Work out the finished part from the listing and answer in its coordinate system (mm). A direction names the side the tool comes from. Round coordinates to 2 decimals unless told otherwise and drop trailing zeros. Loops run counter-clockwise (first coordinate to the right, second up) from the corner with the lowest first, then second, coordinate; pieces in that order, holes last.
from build123d import *

# Parameters (mm, degrees)
SALIENTE_EXTRUIR1_DEPTH = 7
SALIENTE_EXTRUIR2_DEPTH = 30
CORTAR_EXTRUIR3_REACH   = 108.292
CROQUIS3_W              = 3
CROQUIS3_H              = 30
CORTAR_EXTRUIR4_DEPTH   = 7
CROQUIS5_R              = 2
CORTAR_EXTRUIR5_DEPTH   = 5


with BuildPart() as part:
    # Croquis1 → Saliente-Extruir1 (new body)
    with BuildSketch(Plane.XY):
        Polygon((-42.5, 52), (-34.5, 52), (-34.5, 44), (-22.5, 44), (-22.5, 36), (22.5, 36), (22.5, 44), (34.5, 44), (34.5, 52), (42.5, 52), (42.5, -48), (-42.5, -48), align=None)
    extrude(amount=SALIENTE_EXTRUIR1_DEPTH)

    # Croquis2 → Saliente-Extruir2 (add)
    with BuildSketch(Plane.XY.offset(7)):
        Polygon((-42.5, 52), (-42.5, -48), (-34.5, -48), (-34.5, 20), (34.5, 20), (34.5, -48), (42.5, -48), (42.5, 52), (34.5, 52), (34.5, 25), (-34.5, 25), (-34.5, 52), align=None)
    extrude(amount=SALIENTE_EXTRUIR2_DEPTH)

    # Cortar-Extruir3: up to this face of the body (flat: up to its plane)
    cortar_extruir3_end = Plane(part.part.faces().sort_by_distance((42.5, 2, 18.5))[0])
    # Croquis3 → Cortar-Extruir3 (cut, up to the picked face)
    with BuildSketch(Plane.ZY.offset(42.5), mode=Mode.PRIVATE) as cortar_extruir3_sk1:
        with BuildLine():
            Line((37, 52), (7, 52))
            add(Edge.make_bspline(
                [(7, 52), (17.9721482, 28.003586462), (37, 25)],
                knots=[0, 0, 0, 0.777512114, 0.777512114, 0.777512114], degree=2))
            Line((37, 25), (37, 52))
        make_face()
    cortar_extruir3_tool1 = split(extrude(cortar_extruir3_sk1.sketch, amount=-CORTAR_EXTRUIR3_REACH, mode=Mode.PRIVATE), bisect_by=cortar_extruir3_end, keep=Keep.BOTH, mode=Mode.PRIVATE)
    # Croquis3 → Cortar-Extruir3 (cut, up to the picked face)
    with BuildSketch(Plane.ZY.offset(42.5), mode=Mode.PRIVATE) as cortar_extruir3_sk2:
        with BuildLine():
            Line((37, -48), (37, 5))
            add(Edge.make_bspline(
                [(37, 5), (36.935096366, -41.11468491), (12, -48)],
                knots=[0, 0, 0, 0.740176789, 0.740176789, 0.740176789], degree=2))
            Line((12, -48), (37, -48))
        make_face()
    cortar_extruir3_tool2 = split(extrude(cortar_extruir3_sk2.sketch, amount=-CORTAR_EXTRUIR3_REACH, mode=Mode.PRIVATE), bisect_by=cortar_extruir3_end, keep=Keep.BOTH, mode=Mode.PRIVATE)
    # Croquis3 → Cortar-Extruir3 (cut, up to the picked face)
    with BuildSketch(Plane.ZY.offset(42.5), mode=Mode.PRIVATE) as cortar_extruir3_sk3:
        with Locations((16.5, -5)):
            Rectangle(CROQUIS3_W, CROQUIS3_H)
    cortar_extruir3_tool3 = split(extrude(cortar_extruir3_sk3.sketch, amount=-CORTAR_EXTRUIR3_REACH, mode=Mode.PRIVATE), bisect_by=cortar_extruir3_end, keep=Keep.BOTH, mode=Mode.PRIVATE)
    add(cortar_extruir3_tool1.solids().sort_by(Axis((-42.5, 41.293865, 25.499066), (1, 0, 0)))[0], mode=Mode.SUBTRACT)
    add(cortar_extruir3_tool2.solids().sort_by(Axis((-42.5, -37.068003, 30.970324), (1, 0, 0)))[0], mode=Mode.SUBTRACT)
    add(cortar_extruir3_tool3.solids().sort_by(Axis((-42.5, -5, 16.5), (1, 0, 0)))[0], mode=Mode.SUBTRACT)

    # Croquis4 → Cortar-Extruir4 (cut)
    with BuildSketch(Plane.XY.offset(7)):
        Polygon((-13.5, 12.309401077), (-13.5, 7.690598923), (-9.5, 5.381197846), (-5.5, 7.690598923), (-5.5, 12.309401077), (-9.5, 14.618802154), align=None)
        Polygon((-24.5, -10.618802154), (-20.5, -8.309401077), (-20.5, -3.690598923), (-24.5, -1.381197846), (-28.5, -3.690598923), (-28.5, -8.309401077), align=None)
        Polygon((-24.5, 5.381197846), (-20.5, 7.690598923), (-20.5, 12.309401077), (-24.5, 14.618802154), (-28.5, 12.309401077), (-28.5, 7.690598923), align=None)
        Polygon((-24.5, -26.618802154), (-20.5, -24.309401077), (-20.5, -19.690598923), (-24.5, -17.381197846), (-28.5, -19.690598923), (-28.5, -24.309401077), align=None)
        Polygon((-24.5, -42.618802154), (-20.5, -40.309401077), (-20.5, -35.690598923), (-24.5, -33.381197846), (-28.5, -35.690598923), (-28.5, -40.309401077), align=None)
        Polygon((-9.5, -10.618802154), (-5.5, -8.309401077), (-5.5, -3.690598923), (-9.5, -1.381197846), (-13.5, -3.690598923), (-13.5, -8.309401077), align=None)
        Polygon((-9.5, -26.618802154), (-5.5, -24.309401077), (-5.5, -19.690598923), (-9.5, -17.381197846), (-13.5, -19.690598923), (-13.5, -24.309401077), align=None)
        Polygon((-9.5, -42.618802154), (-5.5, -40.309401077), (-5.5, -35.690598923), (-9.5, -33.381197846), (-13.5, -35.690598923), (-13.5, -40.309401077), align=None)
        Polygon((13.5, -40.309401077), (9.5, -42.618802154), (5.5, -40.309401077), (5.5, -35.690598923), (9.5, -33.381197846), (13.5, -35.690598923), align=None)
        Polygon((28.5, -40.309401077), (24.5, -42.618802154), (20.5, -40.309401077), (20.5, -35.690598923), (24.5, -33.381197846), (28.5, -35.690598923), align=None)
        Polygon((28.5, -24.309401077), (24.5, -26.618802154), (20.5, -24.309401077), (20.5, -19.690598923), (24.5, -17.381197846), (28.5, -19.690598923), align=None)
        Polygon((13.5, -24.309401077), (9.5, -26.618802154), (5.5, -24.309401077), (5.5, -19.690598923), (9.5, -17.381197846), (13.5, -19.690598923), align=None)
        Polygon((13.5, -8.309401077), (9.5, -10.618802154), (5.5, -8.309401077), (5.5, -3.690598923), (9.5, -1.381197846), (13.5, -3.690598923), align=None)
        Polygon((28.5, -8.309401077), (24.5, -10.618802154), (20.5, -8.309401077), (20.5, -3.690598923), (24.5, -1.381197846), (28.5, -3.690598923), align=None)
        Polygon((28.5, 7.690598923), (24.5, 5.381197846), (20.5, 7.690598923), (20.5, 12.309401077), (24.5, 14.618802154), (28.5, 12.309401077), align=None)
        Polygon((9.5, 14.618802154), (13.5, 12.309401077), (13.5, 7.690598923), (9.5, 5.381197846), (5.5, 7.690598923), (5.5, 12.309401077), align=None)
    extrude(amount=-CORTAR_EXTRUIR4_DEPTH, mode=Mode.SUBTRACT)

    # Croquis5 → Cortar-Extruir5 (cut)
    with BuildSketch(Plane(origin=(0, 25, 0), x_dir=(1, 0, 0), z_dir=(0, 1, 0))):
        with Locations(Location((0, -22, 0), (0, 0, 270))):
            Circle(CROQUIS5_R)
        with Locations(Location((5, -17, 0), (0, 0, 270))):
            Circle(CROQUIS5_R)
        with Locations(Location((5, -27, 0), (0, 0, 270))):
            Circle(CROQUIS5_R)
        with Locations(Location((-5, -27, 0), (0, 0, 180))):
            Circle(CROQUIS5_R)
        with Locations(Location((-5, -17, 0), (0, 0, 180))):
            Circle(CROQUIS5_R)
        with Locations(Location((15, -17, 0), (0, 0, 270))):
            Circle(CROQUIS5_R)
        with Locations(Location((15, -27, 0), (0, 0, 270))):
            Circle(CROQUIS5_R)
        with Locations(Location((-15, -17, 0), (0, 0, 180))):
            Circle(CROQUIS5_R)
        with Locations(Location((-15, -27, 0), (0, 0, 180))):
            Circle(CROQUIS5_R)
    extrude(amount=-CORTAR_EXTRUIR5_DEPTH, mode=Mode.SUBTRACT)


solid = part.part
Item 1: Section B-B, the plane z = 5.5 is taken. State how many separate pieces and enclosed holes the cut face has, plus the area to 3 significant figures.
Item 2: Each of these flat-tipped pins is pushed along its axis until it touches: P1, Ø6, axis at x = -14, z = 30, coming from the -Y side; P2, Ø21, axis at x = -9, y = 35, coming from the +Z side; P3, Ø2, axis at x = -4.5, y = -4.5, coming from the +Z side; P4, Ø7.5, axis at x = -10.5, z = 4, coming from the +Y side. Where does it stop, or does it pass through?
Item 3: Straight lines are drawn through the part: line 1 (Z direction, x = -15, y = 23.95); line 2 (X direction, y = -3, z = 11); line 3 (X direction, y = 21, z = 22). For each, find the intervals that lie inside material, in ascending order.
Item 4: For faces 1 (the face through (-28.5, -38, 4)), 2 (the face through (-39, -5, 18)), 3 (the face through (42.5, 1, 14)), determine the directions among +Z, -Z, +X, -X, +Y, -Y from which every point of the face is accessible in a straight line to the end or side of a thin tool.
Item 5: Section A-A, the plane x = -15 is taken. Give the vertices of the cut face in (y, z), plus the area to 3 significant figures.
Item 6: Determine the mould class of faces 4 (the face through (17, 23, 17)), 5 (the face through (28.5, 10, 4)) for opening direction Z: pulls with the +Z half, pulls with the -Z half, needs draft (parallel to the pull), parting line crosses it, or undercut.
Answer below:
1. separate pieces: 1
1. enclosed holes: 16
1. area: 6,700 mm2
2. P1: stops at y = 20
2. P2: stops at z = 37
2. P3: stops at z = 7
2. P4: stops at y = 36
3. line 1: z = 0 to 15, 19 to 25, 29 to 37
3. line 2: x = -42.5 to -34.5, 34.5 to 42.5
3. line 3: x = -42.5 to -2, 2 to 42.5
4. face 1: +Z, -Z
4. face 2: +X, -X
4. face 3: +Z, -Z, +X, +Y, -Y
5. outline: (-48, 0) - (36, 0) - (36, 7) - (25, 7) - (25, 15) - (20, 15) - (20, 7) - (-48, 7) - close; (20, 19) - (25, 19) - (25, 25) - (20, 25) - close; (20, 29) - (25, 29) - (25, 37) - (20, 37) - close
5. area: 698 mm2
6. face 4: undercut
6. face 5: needs draft
